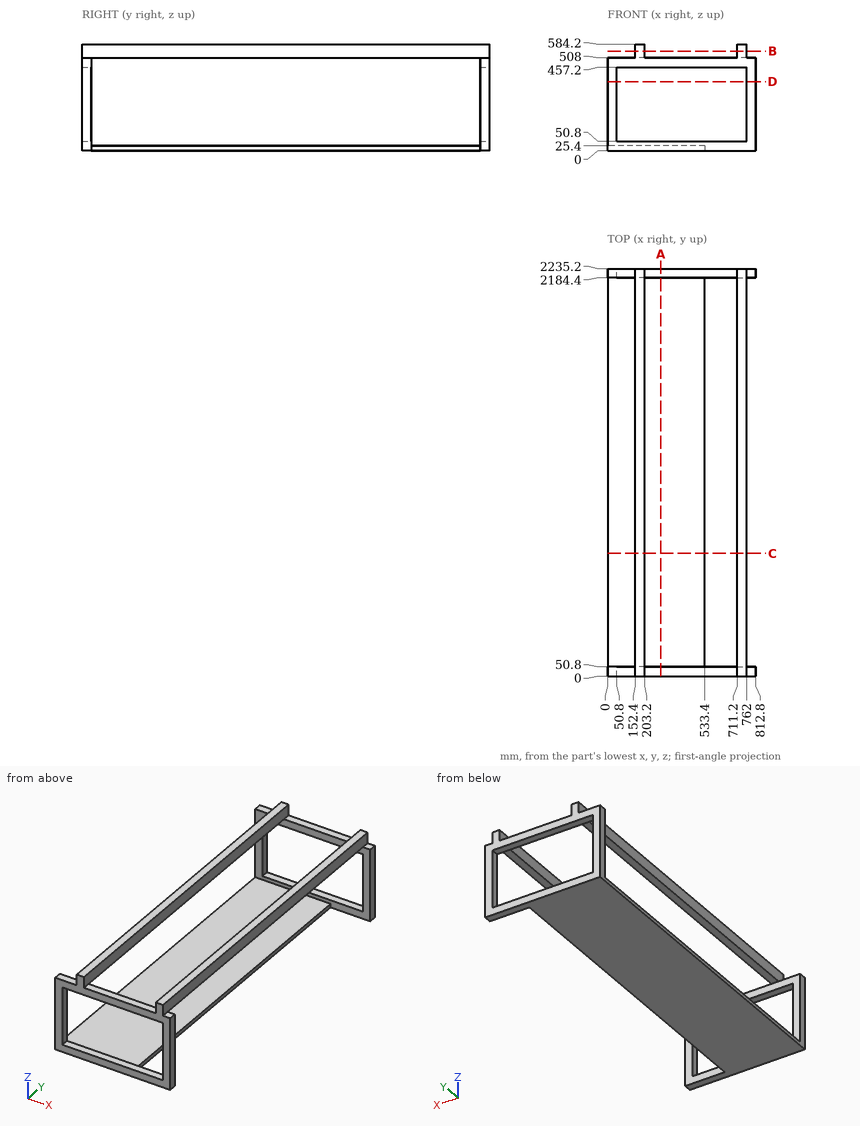
The drawing under review shows one solid part. Ordinate dimensions are in mm from its lowest x, y, z. Coordinates: 2 decimals unless noted, no trailing zeros. Loops run counter-clockwise (first coordinate to the right, second up) from the corner with the lowest first, then second, coordinate; pieces in that order, holes last.
Item 1: Add section B-B (z = 544.5). Write out the cut boundary in (x, y), and give its area (3 significant figures).
Completed:
outline: (152.4, 0) - (203.2, 0) - (203.2, 2235.2) - (152.4, 2235.2) - close; (711.2, 0) - (762, 0) - (762, 2235.2) - (711.2, 2235.2) - close
area: 227,000 mm2
Item 2: Add section A-A (x = 292.5). Write out the cut boundary in (y, z).
Completed:
outline: (0, 0) - (2235.2, 0) - (2235.2, 50.8) - (2184.4, 50.8) - (2184.4, 25.4) - (50.8, 25.4) - (50.8, 50.8) - (0, 50.8) - close; (0, 457.2) - (50.8, 457.2) - (50.8, 508) - (0, 508) - close; (2184.4, 457.2) - (2235.2, 457.2) - (2235.2, 508) - (2184.4, 508) - close
Item 3: Clearance check with flat-ended pins moving along their axes: pin 1 (12 mm diameter, centred on x = 377.5, y = 1584.5, fed in from +Z); pin 2 (8 mm diameter, centred on x = 434, y = 750.5, fed in from -Z); pin 3 (15 mm diameter, centred on x = 544, y = 2197.5, fed in from +Z). State where each tip first meets the part, or that it passes through.
Completed:
pin 1: stops at z = 25.4
pin 2: stops at z = 0
pin 3: stops at z = 508
Item 4: Add section D-D (z = 377.5). Write out the cut boundary in (x, y), and give its area (3 significant figures).
Completed:
outline: (0, 0) - (50.8, 0) - (50.8, 50.8) - (0, 50.8) - close; (0, 2184.4) - (50.8, 2184.4) - (50.8, 2235.2) - (0, 2235.2) - close; (762, 0) - (812.8, 0) - (812.8, 50.8) - (762, 50.8) - close; (762, 2184.4) - (812.8, 2184.4) - (812.8, 2235.2) - (762, 2235.2) - close
area: 10,300 mm2
Item 5: Add section C-C (y = 672). Write out the cut boundary in (x, z).
Completed:
outline: (0, 0) - (533.4, 0) - (533.4, 25.4) - (0, 25.4) - close; (152.4, 508) - (203.2, 508) - (203.2, 584.2) - (152.4, 584.2) - close; (711.2, 508) - (762, 508) - (762, 584.2) - (711.2, 584.2) - close
Item 6: Wall thickness on L1, parallel to Y at x = 320, z = 498.5; L2, parallel to Z at x = 507.5, y = 1426; L3, parallel to Z at x = 724, y = 1607: over which ranges is each line inside the solid? List them lowest first.
Completed:
L1: y = 0 to 50.8, 2184.4 to 2235.2
L2: z = 0 to 25.4
L3: z = 508 to 584.2
